CAD build for the part. Positions are in the model's coordinates, mm. A direction names the side the tool comes from. Coordinates: 2 decimals unless noted, no trailing zeros. Write each loop counter-clockwise with the first axis right and the second up, starting at its lowest first coordinate (ties: lowest second). Pieces come first, ordered by that corner, then holes.
```python
from build123d import *

# Parameters (mm, degrees)
SKETCH1_W                                           = 25
SKETCH1_H                                           = 38
BOSS_EXTRUDE1_DEPTH                                 = 17
CUT_EXTRUDE3_DEPTH                                  = 3.7
CUT_EXTRUDE4_DEPTH                                  = 1.7
CBORE_FOR_6_BINDING_HEAD_MACHINE_SCREW1_D           = 3.7973
CBORE_FOR_6_BINDING_HEAD_MACHINE_SCREW1_CBORE_D     = 7.9375
CBORE_FOR_6_BINDING_HEAD_MACHINE_SCREW1_CBORE_DEPTH = 2.2098
SKETCH12_W                                          = 1
SKETCH12_H                                          = 4.37
SKETCH12_W_2                                        = 6.5
CUT_EXTRUDE5_DEPTH                                  = 2.7
CUT_EXTRUDE6_DEPTH                                  = 4.7


with BuildPart() as part:
    # Sketch1 → Boss-Extrude1 (new body)
    with BuildSketch(Plane(origin=(0, 0, 0), x_dir=(1, 0, 0), z_dir=(0, 1, 0))):
        with Locations((-18481.446731235, 11298.191283293)):
            Rectangle(SKETCH1_W, SKETCH1_H)
    extrude(amount=BOSS_EXTRUDE1_DEPTH)

    # Sketch2 → Cut-Extrude3 (cut)
    with BuildSketch(Plane(origin=(0, 17, 0), x_dir=(1, 0, 0), z_dir=(0, 1, 0))):
        with BuildLine():
            Line((-18493.946731235, 11291.191283293), (-18489.946731235, 11291.191283293))
            ThreePointArc((-18489.946731235, 11291.191283293), (-18488.532517672, 11291.777069731), (-18487.946731235, 11293.191283293))
            Line((-18487.946731235, 11293.191283293), (-18487.946731235, 11303.191283293))
            ThreePointArc((-18487.946731235, 11303.191283293), (-18488.532517672, 11304.605496855), (-18489.946731235, 11305.191283293))
            Line((-18489.946731235, 11305.191283293), (-18493.946731235, 11305.191283293))
            Line((-18493.946731235, 11305.191283293), (-18493.946731235, 11291.191283293))
        make_face()
    extrude(amount=-CUT_EXTRUDE3_DEPTH, mode=Mode.SUBTRACT)

    # Sketch2<6> → Cut-Extrude4 (cut)
    with BuildSketch(Plane(origin=(0, 17, 0), x_dir=(1, 0, 0), z_dir=(0, 1, 0))):
        with BuildLine():
            Line((-18475.446731235, 11301.191283293), (-18475.446731235, 11295.191283293))
            ThreePointArc((-18475.446731235, 11295.191283293), (-18474.860944797, 11293.777069731), (-18473.446731235, 11293.191283293))
            Line((-18473.446731235, 11293.191283293), (-18468.946731235, 11293.191283293))
            Line((-18468.946731235, 11293.191283293), (-18468.946731235, 11303.191283293))
            Line((-18468.946731235, 11303.191283293), (-18473.446731235, 11303.191283293))
            ThreePointArc((-18473.446731235, 11303.191283293), (-18474.860944797, 11302.605496855), (-18475.446731235, 11301.191283293))
        make_face()
    extrude(amount=-CUT_EXTRUDE4_DEPTH, mode=Mode.SUBTRACT)

    # CBORE for #6 Binding Head Machine Screw1 (through all)
    with Locations(Plane(origin=(0, 17, 0), x_dir=(1, 0, 0), z_dir=(0, 1, 0))):
        with Locations((-18488.946731235, 11310.191283293), (-18473.946731235, 11310.191283293), (-18473.946731235, 11286.191283293), (-18488.946731235, 11286.191283293)):
            CounterBoreHole(CBORE_FOR_6_BINDING_HEAD_MACHINE_SCREW1_D / 2, CBORE_FOR_6_BINDING_HEAD_MACHINE_SCREW1_CBORE_D / 2, CBORE_FOR_6_BINDING_HEAD_MACHINE_SCREW1_CBORE_DEPTH)

    # Sketch12 → Cut-Extrude5 (cut)
    with BuildSketch(Plane(origin=(0, 17, 0), x_dir=(1, 0, 0), z_dir=(0, 1, 0))):
        with BuildLine():
            Line((-18476.446731235, 11300.376283293), (-18476.446731235, 11296.006283293))
            ThreePointArc((-18476.446731235, 11296.006283293), (-18478.631731235, 11298.191283293), (-18476.446731235, 11300.376283293))
        make_face()
        with Locations((-18475.946731235, 11298.191283293)):
            Rectangle(SKETCH12_W, SKETCH12_H)
        with Locations((-18472.196731235, 11298.191283293)):
            Rectangle(SKETCH12_W_2, SKETCH12_H)
    extrude(amount=-CUT_EXTRUDE5_DEPTH, mode=Mode.SUBTRACT)

    # Sketch13 → Cut-Extrude6 (cut)
    with BuildSketch(Plane(origin=(0, 17, 0), x_dir=(1, 0, 0), z_dir=(0, 1, 0))):
        with BuildLine():
            ThreePointArc((-18486.936731235, 11303.441283293), (-18483.853745669, 11302.164268859), (-18482.576731235, 11299.081283293))
            Line((-18482.576731235, 11299.081283293), (-18482.576731235, 11297.301283293))
            ThreePointArc((-18482.576731235, 11297.301283293), (-18483.853745669, 11294.218297727), (-18486.936731235, 11292.941283293))
            Line((-18486.936731235, 11292.941283293), (-18486.946731235, 11292.941283293))
            Line((-18486.946731235, 11292.941283293), (-18486.946731235, 11303.441283293))
            Line((-18486.946731235, 11303.441283293), (-18486.936731235, 11303.441283293))
        make_face()
        with BuildLine():
            ThreePointArc((-18487.946731235, 11303.191283293), (-18487.950656716, 11303.316529118), (-18487.962417752, 11303.441283293))
            Line((-18487.962417752, 11303.441283293), (-18493.946731235, 11303.441283293))
            Line((-18493.946731235, 11303.441283293), (-18493.946731235, 11292.941283293))
            Line((-18493.946731235, 11292.941283293), (-18487.962417752, 11292.941283293))
            ThreePointArc((-18487.962417752, 11292.941283293), (-18487.950656716, 11293.066037468), (-18487.946731235, 11293.191283293))
            Line((-18487.946731235, 11293.191283293), (-18487.946731235, 11303.191283293))
        make_face()
        with BuildLine():
            Line((-18486.946731235, 11292.941283293), (-18486.946731235, 11303.441283293))
            Line((-18486.946731235, 11303.441283293), (-18487.962417752, 11303.441283293))
            ThreePointArc((-18487.962417752, 11303.441283293), (-18487.950656716, 11303.316529118), (-18487.946731235, 11303.191283293))
            Line((-18487.946731235, 11303.191283293), (-18487.946731235, 11293.191283293))
            ThreePointArc((-18487.946731235, 11293.191283293), (-18487.950656716, 11293.066037468), (-18487.962417752, 11292.941283293))
            Line((-18487.962417752, 11292.941283293), (-18486.946731235, 11292.941283293))
        make_face()
    extrude(amount=-CUT_EXTRUDE6_DEPTH, mode=Mode.SUBTRACT)


solid = part.part
```
Item 1: Saw through at D-D, the plane z = -11298.5. Write the cut outline in (x, y), and give its area (3 significant figures).
Item 2: Saw through at B-B, the plane y = 5. Write the cut outline in (x, z), and give its area (3 significant figures).
Item 3: Wall check: line 1 along Z through (x, y) = (-18488.75, 12.75); line 2 along Z through (x, y) = (-18475.25, 16); line 3 along X through (y, z) = (15.75, -11313.5). Give the ranges that are in metal, low to high.
Item 4: Two-plate mould, pull along Z, no slides. Class faces 5 (the flat face through (-18472, 14.79, -11311)), 6 (the flat face through (-18493.947, 8, -11298)), 7 (the flat face through (-18471, 16, -11303.191)): +Z half, -Z half, draft (parallel to the pull), parting line (faces both ways), or undercut.
Item 5: Saw through at C-C, the plane x = -18483. Write the cut outline in (y, z), and give its area (3 significant figures).
Item 6: Flat gauge pins, fed straight in: pin 1 Ø0.5 at (y, z) = (13.5, -11298.5) entering from -X; pin 2 Ø2.5 at (x, z) = (-18473, -11295) entering from +Y; pin 3 Ø4 at (x, z) = (-18489, -11285) entering from +Y. Where does each tip first touch, or does it go through?
Item 7: Which spindle directions (+Z, -Z, +X, -X, +Y, -Y) get a long thin tool onto all of the face, cutting with end or side? Do faces 1 (the cylindrical face through (-18472.44, 7.292, -11285.036)), 2 (the flat face through (-18487, 14.79, -11287)), 3 (the flat face through (-18492, 15, -11305.191)), 4 (the flat face through (-18474, 15, -11296.006)). Say none if no direction does.
Item 8: Saw through at A-A, the plane z = -11311.5. Write the cut outline in (x, y).
Working result:
1. outline: (-18493.95, 0) - (-18468.95, 0) - (-18468.95, 14.3) - (-18478.61, 14.3) - (-18478.61, 17) - (-18482.58, 17) - (-18482.58, 12.3) - (-18493.95, 12.3) - close
1. area: 345 mm2
2. outline: (-18493.95, -11317.19) - (-18468.95, -11317.19) - (-18468.95, -11279.19) - (-18493.95, -11279.19) - close; hole circle Ø3.8 at (-18488.95, -11310.19); hole circle Ø3.8 at (-18488.95, -11286.19); hole circle Ø3.8 at (-18473.95, -11310.19); hole circle Ø3.8 at (-18473.95, -11286.19)
2. area: 905 mm2
3. line 1: z = -11317.19 to -11312.08, -11308.3 to -11303.44, -11292.94 to -11288.08, -11284.3 to -11279.19
3. line 2: z = -11317.19 to -11313.94, -11306.44 to -11302.06, -11294.33 to -11289.94, -11282.44 to -11279.19
3. line 3: x = -18493.95 to -18491.14, -18486.76 to -18476.14, -18471.76 to -18468.95
4. face 5: undercut
4. face 6: draft
4. face 7: undercut
5. outline: (0, -11317.19) - (17, -11317.19) - (17, -11300.96) - (12.3, -11300.96) - (12.3, -11295.43) - (17, -11295.43) - (17, -11279.19) - (0, -11279.19) - close
5. area: 620 mm2
6. pin 1: stops at x = -18482.58
6. pin 2: stops at y = 15.3
6. pin 3: stops at y = 14.79
7. face 1: +Y, -Y
7. face 2: +Y
7. face 3: -X, +Y
7. face 4: +X, +Y
8. outline: (-18493.95, 0) - (-18490.32, 0) - (-18490.32, 14.79) - (-18492.69, 14.79) - (-18492.69, 17) - (-18493.95, 17) - close; (-18487.57, 0) - (-18475.32, 0) - (-18475.32, 14.79) - (-18477.69, 14.79) - (-18477.69, 17) - (-18485.2, 17) - (-18485.2, 14.79) - (-18487.57, 14.79) - close; (-18472.57, 0) - (-18468.95, 0) - (-18468.95, 17) - (-18470.2, 17) - (-18470.2, 14.79) - (-18472.57, 14.79) - close
